Print and shaded views of the part. All mm, measured from the part's lowest x, y and z. A direction names the side the tool comes from. Round coordinates to 2 decimals unless told otherwise and drop trailing zeros. Write each loop counter-clockwise with the first axis right and the second up, starting at its lowest first coordinate (ties: lowest second). Pieces come first, ordered by that corner, then holes.
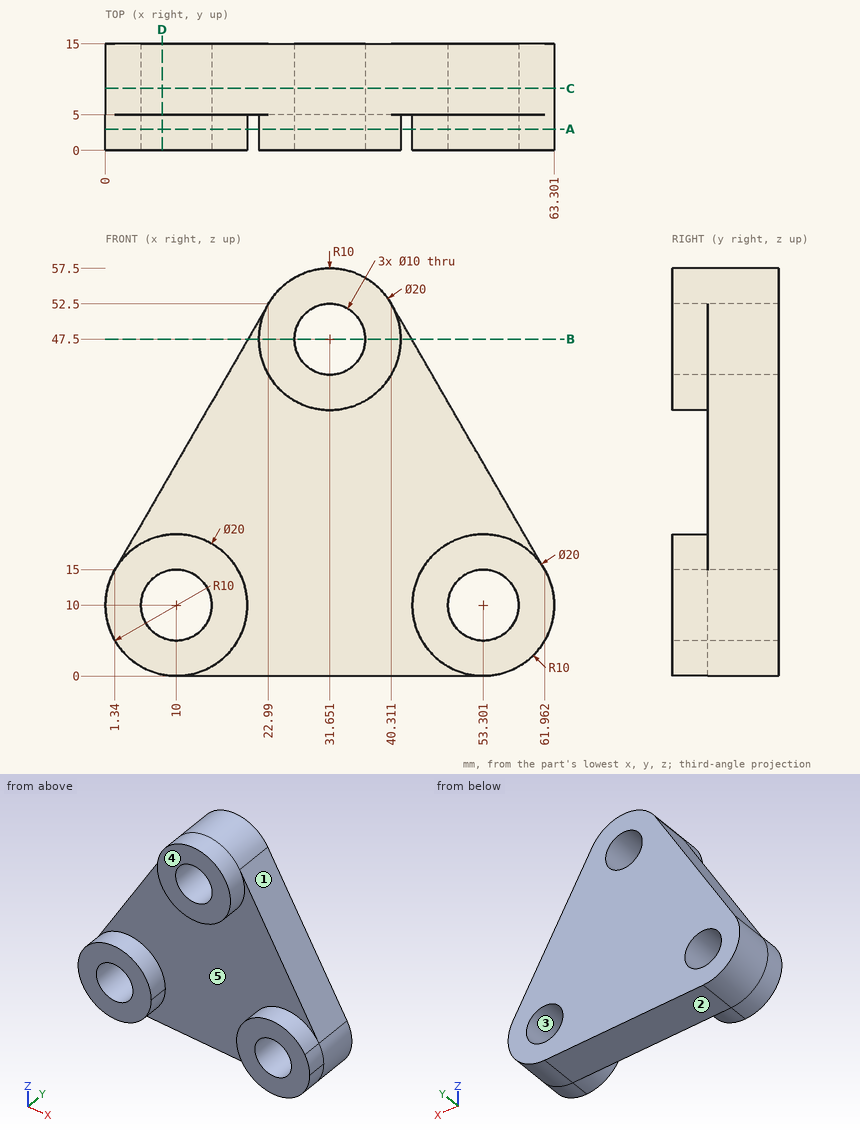
1) Slice it at B-B (z = 47.5). Write the cut outline in (x, y), plus the area to 3 significant figures.
Results:
outline: (20.1, 5) - (21.65, 5) - (21.65, 0) - (26.65, 0) - (26.65, 15) - (20.1, 15) - close; (36.65, 0) - (41.65, 0) - (41.65, 5) - (43.2, 5) - (43.2, 15) - (36.65, 15) - close
area: 181 mm2
2) Slice it at C-C (y = 8.75). Write the cut outline in (x, z), plus the area to 3 significant figures.
Results:
outline: (1.34, 15) arc R10 ccw to (10, 0) - (53.3, 0) arc R10 ccw to (61.96, 15) - (40.31, 52.5) arc R10 ccw to (22.99, 52.5) - close; hole circle Ø10 at (10, 10); hole circle Ø10 at (31.65, 47.5); hole circle Ø10 at (53.3, 10)
area: 2,190 mm2
3) Slice it at D-D (x = 8). Write the cut outline in (y, z) (1 decimal).
Results:
outline: (0, 0.2) - (15, 0.2) - (15, 5.4) - (0, 5.4) - close; (0, 14.6) - (15, 14.6) - (15, 26.5) - (5, 26.5) - (5, 19.8) - (0, 19.8) - close
4) Mould opens along X. For the marked faces 1, 2 and 3 say: released by +X, released by -X, zero draft, split by the parting line, or undercut.
Results:
face 1: released by +X
face 2: zero draft
face 3: undercut
5) Which spindle directions (+Z, -Z, +X, -X, +Y, -Y) get a long thin tool onto all of the face, cutting with end or side? Do the marked faces 4 and 5. Say none if no direction does.
Results:
face 4: +Z, -Z, +X, -X, -Y
face 5: -Y
6) Wall check: L1, parallel to X at y = 11.25, z = 12 (1 decimal); L2, parallel to Y at x = 54.5, z = 23.5; L3, parallel to X at y = 3.5, z = 45 (1 decimal). Give the ranges that are in metal, low to high.
Results:
L1: x = 0.2 to 5.4, 14.6 to 48.7, 57.9 to 63.1
L2: y = 5 to 15
L3: x = 22 to 27.3, 36 to 41.3
7) Slice it at A-A (y = 3). Write the cut outline in (x, z), plus the area to 3 significant figures.
Results:
outline: circle Ø20 at (10, 10); circle Ø20 at (31.65, 47.5); circle Ø20 at (53.3, 10); hole circle Ø10 at (10, 10); hole circle Ø10 at (31.65, 47.5); hole circle Ø10 at (53.3, 10)
area: 707 mm2
8) Pin check, flat tips, straight feed: pin 1 Ø3 at (x, y) = (34.5, 2.5) entering from +Z; pin 2 Ø16 at (x, z) = (53.3, 10) entering from -Y; pin 3 Ø3 at (y, z) = (3, 43.5) entering from -X. Stop position of each tip, or through.
Results:
pin 1: stops at z = 57.41
pin 2: stops at y = 0
pin 3: stops at x = 21.97
